Job drawing, mm, ordinate dimensions from the low corner. One solid piece. Coordinates: 2 decimals unless noted, no trailing zeros. Loops run counter-clockwise (first coordinate to the right, second up) from the corner with the lowest first, then second, coordinate; pieces in that order, holes last. Notation, with made-up numbers: M 63,53.25 L 94,53.25 A23 cw 94,87.25 Z; hole C -40,6 d6. An arc over 180 degrees is marked long. Answer as a JSON object with one key per item and string values. Group by question number.
1. Saw through at A-A on z = 7.25. Write the cut outline in (x, y), then the cut area to 3 significant figures.
2. Mould opens along X. For the marked faces 1 and 2 say: released by +X, released by -X, zero draft, split by the parting line, or undercut.
3. Drill centre lines: L1, parallel to Y at x = 95, z = 9.5; L2, parallel to X at y = 89.5, z = 13.5; L3, parallel to Z at x = 194, y = 35. Where is each one in solid material? Low to high.
4. Saw through at C-C on y = 143. Write the cut outline in (x, z), then the cut area to 4 significant figures.
5. Saw through at B-B on x = 168. Write the cut outline in (y, z).
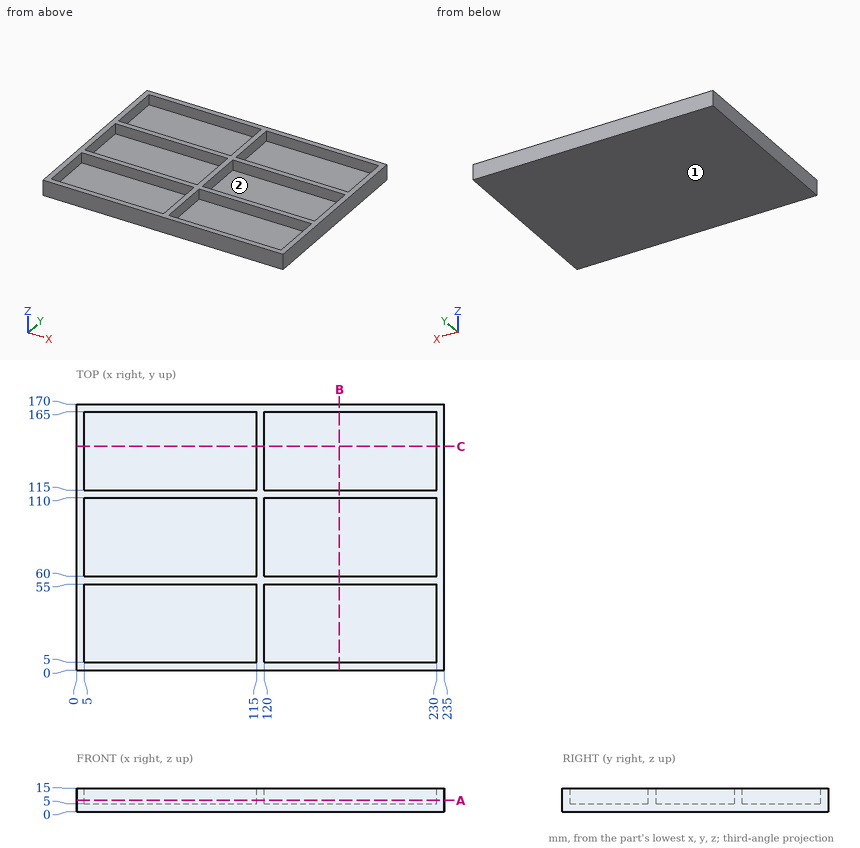
Outcome:
{
 "1": {"outline": "M 0,0 L 235,0 L 235,170 L 0,170 Z; hole M 5,5 L 115,5 L 115,55 L 5,55 Z; hole M 5,60 L 115,60 L 115,110 L 5,110 Z; hole M 5,115 L 115,115 L 115,165 L 5,165 Z; hole M 120,5 L 230,5 L 230,55 L 120,55 Z; hole M 120,60 L 230,60 L 230,110 L 120,110 Z; hole M 120,115 L 230,115 L 230,165 L 120,165 Z", "area": "6,950 mm²"},
 "2": {"face 1": "zero draft", "face 2": "undercut"},
 "3": {"L1": "y = 0 to 5, 55 to 60, 110 to 115, 165 to 170", "L2": "x = 0 to 5, 115 to 120, 230 to 235", "L3": "z = 0 to 5"},
 "4": {"outline": "M 0,0 L 235,0 L 235,15 L 230,15 L 230,5 L 120,5 L 120,15 L 115,15 L 115,5 L 5,5 L 5,15 L 0,15 Z", "area": "1,325 mm²"},
 "5": {"outline": "M 0,0 L 170,0 L 170,15 L 165,15 L 165,5 L 115,5 L 115,15 L 110,15 L 110,5 L 60,5 L 60,15 L 55,15 L 55,5 L 5,5 L 5,15 L 0,15 Z"}
}
